Can you work these out from the model? Positions are in its coordinate system, mm. Give positions to 0.01 mm unless a question says otherwise; leave off trailing zeros. Order: outer loops, then holes, each group sorted by start corner. A loop starts at its lowest first (then second) coordinate and runs counter-clockwise, first axis right, second up.
Item 1: I want a section at A-A, the plane y = 93.5. Write out the boundary of the cut face in (x, z), then the cut area to 3 significant figures.
Item 2: If I drill on line 1 along Y through (x, z) = (0, 8.65); line 2 along Y through (x, z) = (8.65, 0); line 3 along Z through (x, y) = (-0.5, -39), over which ranges is the centre line in solid material (lowest first)?
Item 3: I'm going to push flat-ended pins straight in: pin 1 Ø2.5 at (x, y) = (0, 200) entering from +Z; pin 2 Ø2 at (x, y) = (-7.5, -26.5) entering from +Z; pin 3 Ø1 at (y, z) = (191.5, -3.5) entering from -X; pin 4 Ø8 at (y, z) = (-75, -7.5) entering from +X. Where does each tip first touch, or does it pass through?
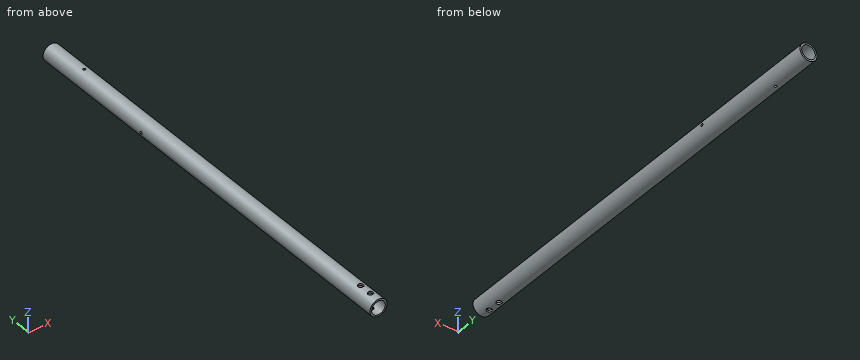
Solid Edge part; units mm, degrees
sketch "Sketch1" plane through (0, 0, 0) normal (0, -1, 0) x (1, 0, 0)
  circle A0 centre (0, 0) radius 10
  circle A1 centre (0, 0) radius 8
extrude "Protrusion1" add sketch "Sketch1" along normal mid plane 500
sketch "Sketch2" plane through (0, 0, 0) normal (0, 0, 1) x (1, 0, 0)
  circle A0 centre (0, -238) radius 3
  circle A1 centre (0, -223) radius 3
extrude "ExtrudedCutout_1" cut sketch "Sketch2" along normal mid plane 103.8089
sketch "Sketch3" plane through (0, 0, 0) normal (1, 0, 0) x (0, 1, 0)
  circle A0 centre (100, 0) radius 1.5
extrude "ExtrudedCutout_3" cut sketch "Sketch3" along normal mid plane 217.8722
sketch "Sketch4" plane through (0, 0, 0) normal (0, 0, 1) x (1, 0, 0)
  circle A0 centre (0, 200) radius 1.5
extrude "ExtrudedCutout_4" cut sketch "Sketch4" along normal mid plane 490.2317
properties material "PVC"
Results list:
1. outline: circle Ø20 at (0, 0); hole circle Ø16 at (0, 0)
1. area: 113 mm2
2. line 1: y = -250 to -241, -235 to -226, -220 to 198.5, 201.5 to 250
2. line 2: y = -250 to 98.5, 101.5 to 250
2. line 3: z = -9.99 to -7.98, 7.98 to 9.99
3. pin 1: passes through
3. pin 2: stops at z = 7.6
3. pin 3: stops at x = -9.54
3. pin 4: stops at x = 9.37
